from build123d import *

# Parameters (mm, degrees)
EXTRUDE_1_DEPTH     = 6
CUT_EXTRUDE_3_REACH = 8
SKETCH_2_R          = 2
SKETCH_2_W          = 8
SKETCH_2_H          = 2
CHAMFER_1_SIZE      = 3


with BuildPart() as part:
    # 草图1 → 凸台-拉伸1 (new body)
    with BuildSketch(Plane(origin=(0, 0, 0), x_dir=(1, 0, 0), z_dir=(0, 1, 0))):
        Polygon((-4, 5), (-4, 10), (-10, 10), (-10, 5), (-10, 0), (10, 0), (10, 5), (10, 10), (4, 10), (4, 5), align=None)
    extrude(amount=EXTRUDE_1_DEPTH)

    # 草图2 → 切除-拉伸3 (cut, up to next)
    with BuildSketch(Plane(origin=(0, 6, 0), x_dir=(1, 0, 0), z_dir=(0, 1, 0)), mode=Mode.PRIVATE) as cut_extrude_3_sk1:
        with Locations((-7, 7)):
            Circle(SKETCH_2_R)
    cut_extrude_3_tool1 = extrude(cut_extrude_3_sk1.sketch, amount=-CUT_EXTRUDE_3_REACH, mode=Mode.PRIVATE) & part.part
    add(cut_extrude_3_tool1.solids().sort_by_distance((-7, 6, -7))[0], mode=Mode.SUBTRACT)
    # 草图2 → 切除-拉伸3 (cut, up to next)
    with BuildSketch(Plane(origin=(0, 6, 0), x_dir=(1, 0, 0), z_dir=(0, 1, 0)), mode=Mode.PRIVATE) as cut_extrude_3_sk2:
        with Locations((7, 7)):
            Circle(SKETCH_2_R)
    cut_extrude_3_tool2 = extrude(cut_extrude_3_sk2.sketch, amount=-CUT_EXTRUDE_3_REACH, mode=Mode.PRIVATE) & part.part
    add(cut_extrude_3_tool2.solids().sort_by_distance((7, 6, -7))[0], mode=Mode.SUBTRACT)
    # 草图2 → 切除-拉伸3 (cut, up to next)
    with BuildSketch(Plane(origin=(0, 6, 0), x_dir=(1, 0, 0), z_dir=(0, 1, 0)), mode=Mode.PRIVATE) as cut_extrude_3_sk3:
        with Locations((0, 2)):
            Rectangle(SKETCH_2_W, SKETCH_2_H)
    cut_extrude_3_tool3 = extrude(cut_extrude_3_sk3.sketch, amount=-CUT_EXTRUDE_3_REACH, mode=Mode.PRIVATE) & part.part
    add(cut_extrude_3_tool3.solids().sort_by_distance((0, 6, -2))[0], mode=Mode.SUBTRACT)

    # 倒角1
    chamfer_1_edges = [part.edges().sort_by_distance(p)[0] for p in [
        (10, 3, 0),
        (-10, 3, 0),
    ]]
    chamfer(chamfer_1_edges, length=CHAMFER_1_SIZE)


solid = part.part
Work out the finished part from the listing and answer in its coordinate system (mm). A direction names the side the tool comes from. Coordinates: 2 decimals unless noted, no trailing zeros. Write each loop counter-clockwise with the first axis right and the second up, starting at its lowest first coordinate (ties: lowest second). Pieces come first, ordered by that corner, then holes.
1. The part is cut by section A-A, the plane z = -7. Write down the section's boundary in (x, y), and give its area (3 significant figures).
Results list:
outline: (-10, 0) - (-9, 0) - (-9, 6) - (-10, 6) - close; (-5, 0) - (-4, 0) - (-4, 6) - (-5, 6) - close; (4, 0) - (5, 0) - (5, 6) - (4, 6) - close; (9, 0) - (10, 0) - (10, 6) - (9, 6) - close
area: 24.0 mm2
2. Consider line 1 along X through (y, z) = (2.75, -7); line 2 along X through (y, z) = (4.9, -9.5); line 3 along X through (y, z) = (4.65, -8.5). Determine where each line is inside the solid, lowest interval first.
Results list:
line 1: x = -10 to -9, -5 to -4, 4 to 5, 9 to 10
line 2: x = -10 to -4, 4 to 10
line 3: x = -10 to -8.32, -5.68 to -4, 4 to 5.68, 8.32 to 10
3. For faces 1 (the flat face through (-4, 3, -7)), 2 (the flat face through (7, 3, -10)), 3 (the flat face through (0, 3, -3)), determine the directions among +Z, -Z, +X, -X, +Y, -Y from which every point of the face is accessible in a straight line to the end or side of a thin tool.
Results list:
face 1: -Z, +Y, -Y
face 2: -Z, +X, -X, +Y, -Y
face 3: +Y, -Y
4. The part is cut by section B-B, the plane y = 4.65. Write down the section's boundary in (x, z).
Results list:
outline: (-10, -10) - (-4, -10) - (-4, -5) - (4, -5) - (4, -10) - (10, -10) - (10, -3) - (7, 0) - (-7, 0) - (-10, -3) - close; hole circle Ø4 at (-7, -7); hole (-4, -3) - (4, -3) - (4, -1) - (-4, -1) - close; hole circle Ø4 at (7, -7)
5. Flat-ended cylindrical pins translate along their axes: pin 1 (1.6 mm diameter, centred on y = 2.5, z = -2.5, fed in from +X); pin 2 (2 mm diameter, centred on y = 3.5, z = -1.5, fed in from -X); pin 3 (3 mm diameter, centred on x = 1, y = 4, fed in from -Z). Find the tip coordinate at first contact, or state that the pin passes through.
Results list:
pin 1: stops at x = 10
pin 2: stops at x = -9.5
pin 3: stops at z = -5
6. For a pull along X with two mould halves and no side action, classify faces 4 (the flat face through (0, 3, 0)), 5 (the flat face through (9, 3, -2)), 6 (the cylindrical face through (5.526, 3.042, -8.352)), 7 (the flat face through (-10, 3, -7)) as +X half, -X half, draft (parallel to the pull), parting line (faces both ways), or undercut.
Results list:
face 4: draft
face 5: +X half
face 6: undercut
face 7: -X half
7. The part is cut by section D-D, the plane z = -2.5. Write down the section's boundary in (x, y), and give its area (3 significant figures).
Results list:
outline: (-9.5, 0) - (-4, 0) - (-4, 6) - (-9.5, 6) - close; (4, 0) - (9.5, 0) - (9.5, 6) - (4, 6) - close
area: 66.0 mm2
8. The part is cut by section C-C, the plane x = 0.25. Write down the section's boundary in (y, z).
Results list:
outline: (0, -5) - (6, -5) - (6, -3) - (0, -3) - close; (0, -1) - (6, -1) - (6, 0) - (0, 0) - close
